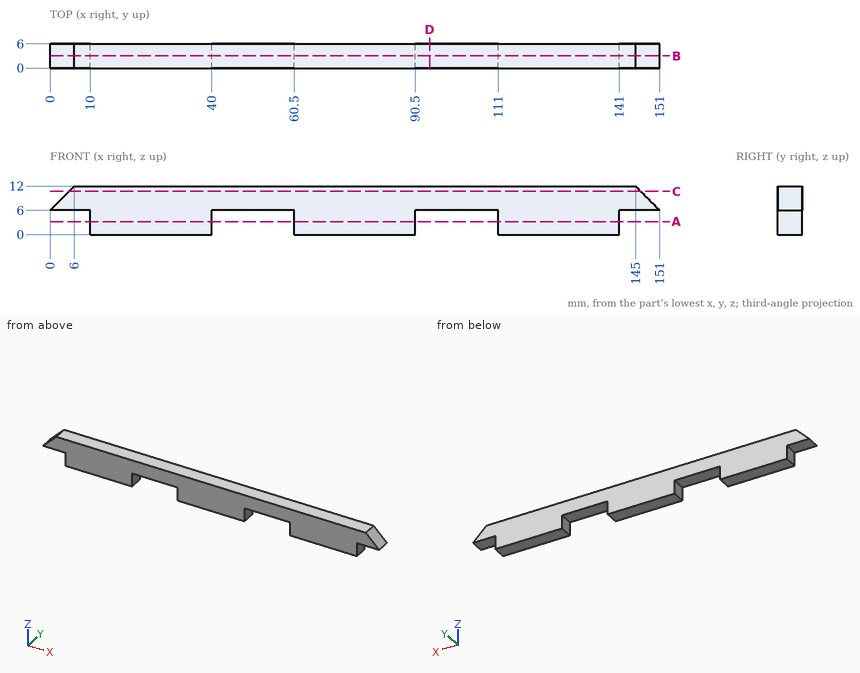
Study the drawing (mm; zero at the part's minimum x, y, z) and answer. Give positions to 0.01 mm unless a question says otherwise; leave off trailing zeros. Loops run counter-clockwise (first coordinate to the right, second up) from the corner with the lowest first, then second, coordinate; pieces in that order, holes last. Notation, with made-up numbers: (7.25, 84) -> (49.25, 84) arc R6 cw to (49.25, 94) -> close; hole circle Ø3 at (54.5, 15.5). An arc over 180 degrees is marked (long way). Use a Markdown table: item, result. Add a question column.
1) Each of these flat-tipped pins is pushed along its axis until it touches: P1, Ø3, axis at y = 3, z = 1.5, coming from the -X side; P2, Ø3, axis at x = 146.5, y = 1.5, coming from the -Z side; P3, Ø2, axis at y = 1.5, z = 10, coming from the +X side. Where does it stop, or does it pass through?
2) The part is cut by section D-D, the plane x = 94. Determine the outline of the cut face in (y, z).
3) The part is cut by section C-C, the plane z = 10.75. Determine the outline of the cut face in (x, y), plus the area to 3 significant figures.
4) Consider line 1 along X through (y, z) = (4.95, 1.25); line 2 along Z through (x, y) = (94, 0.65); line 3 along X through (y, z) = (3.6, 11.25). Determine where each line is inside the solid, lowest interval first.
5) The part is cut by section B-B, the plane y = 3.05. Determine the outline of the cut face in (x, z).
6) The part is cut by section A-A, the plane z = 3.25. Determine the outline of the cut face in (x, y), plus the area to 3 significant figures.
Reported:
| question | item | result |
|---|---|---|
| 1 | P1 | stops at x = 10 |
| 1 | P2 | stops at z = 6 |
| 1 | P3 | stops at x = 148 |
| 2 | outline | (0, 6) -> (6, 6) -> (6, 12) -> (0, 12) -> close |
| 3 | outline | (4.75, 0) -> (146.25, 0) -> (146.25, 6) -> (4.75, 6) -> close |
| 3 | area | 849 mm^2 |
| 4 | line 1 | x = 10 to 40, 60.5 to 90.5, 111 to 141 |
| 4 | line 2 | z = 6 to 12 |
| 4 | line 3 | x = 5.25 to 145.75 |
| 5 | outline | (0, 6) -> (10, 6) -> (10, 0) -> (40, 0) -> (40, 6) -> (60.5, 6) -> (60.5, 0) -> (90.5, 0) -> (90.5, 6) -> (111, 6) -> (111, 0) -> (141, 0) -> (141, 6) -> (151, 6) -> (145, 12) -> (6, 12) -> close |
| 6 | outline | (10, 0) -> (40, 0) -> (40, 6) -> (10, 6) -> close; (60.5, 0) -> (90.5, 0) -> (90.5, 6) -> (60.5, 6) -> close; (111, 0) -> (141, 0) -> (141, 6) -> (111, 6) -> close |
| 6 | area | 540 mm^2 |
